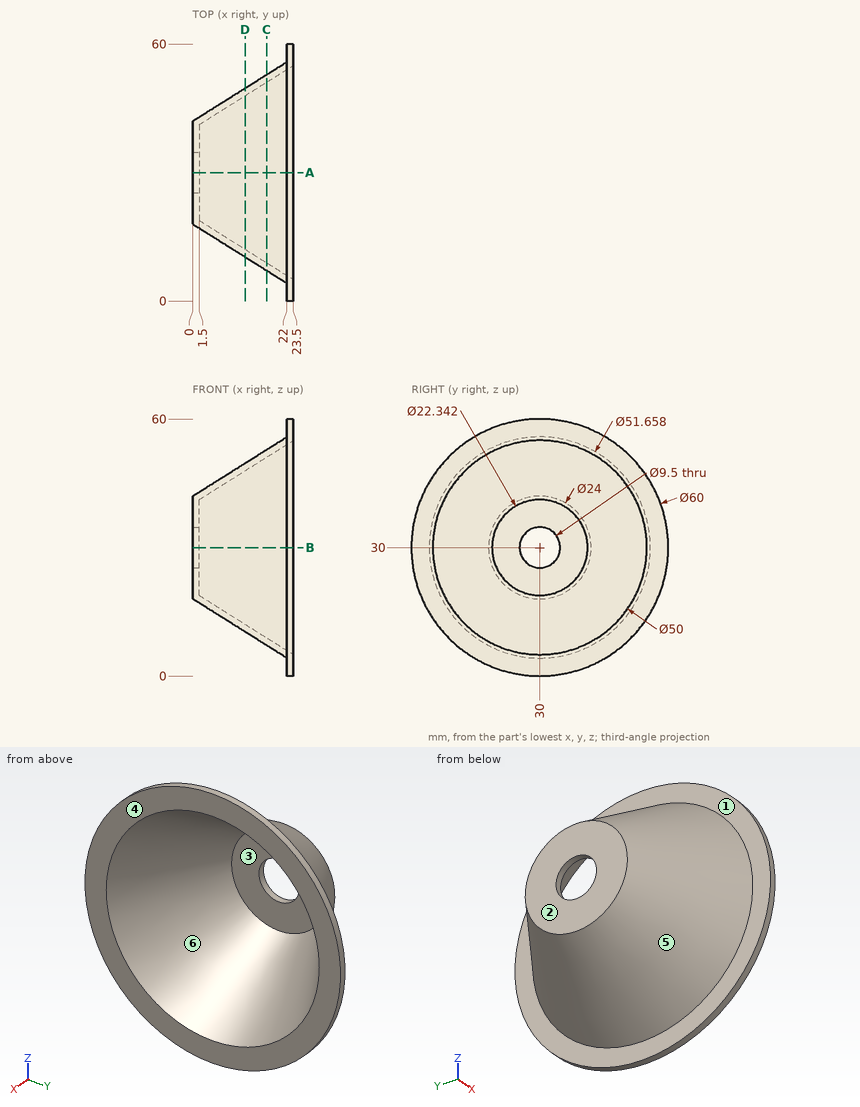
Part print with two shaded views. Sizes in mm from the minimum x, y, z corner. A direction names the side the tool comes from. Coordinates: 2 decimals unless noted, no trailing zeros. Write each loop counter-clockwise with the first axis right and the second up, starting at its lowest first coordinate (ties: lowest second). Pieces come first, ordered by that corner, then holes. Notation, with made-up numbers: (-8, 4) - (14, 4) arc R8 ccw to (14, 14) - close; hole circle Ø1 at (78, -8). An arc over 180 degrees is marked (long way). Use a Markdown table: item, result. Add a question column.
Item 1: Drop flat-ended pins along their axis: pin 1 (10 mm diameter, centred on x = 17.5, y = 52.5, fed in from -Z); pin 2 (12 mm diameter, centred on y = 51.5, z = 10.5, fed in from -X); pin 3 (10 mm diameter, centred on y = 41.5, z = 35, fed in from +X). Give the stop position or say it passes through.
Item 2: Band-saw the part on D-D, the plane x = 12.25. Write the cut outline in (y, z).
Item 3: 3-axis set-ups, long thin cutter, end or side, ignore diameter. For the marked faces 1 and 2: which of +Z, -Z, +X, -X, +Y, -Y reach the whole face in a straight line?
Item 4: Band-saw the part on C-C, the plane x = 17.25. Write the cut outline in (y, z).
Item 5: Drill centre lines: line 1 along X through (y, z) = (48, 8.5); line 2 along Y through (x, z) = (15.5, 24); line 3 along Y through (x, z) = (0.45, 30). Where is each one in solid material? Low to high.
Item 6: Band-saw the part on A-A, the plane y = 30. Write the cut outline in (x, z), and give its area (3 significant figures).
Item 7: Two-plate mould, pull along Z, no slides. Class the marked faces 3, 4, 5 and 6: pulls with the +Z half, pulls with the -Z half, needs draft (parallel to the pull), parting line crosses it, or undercut.
A:
| question | item | result |
|---|---|---|
| 1 | pin 1 | stops at z = 7.93 |
| 1 | pin 2 | stops at x = 17.54 |
| 1 | pin 3 | stops at x = 11.63 |
| 2 | outline | circle Ø39.4 at (30, 30); hole circle Ø35.86 at (30, 30) |
| 3 | face 1 | -X |
| 3 | face 2 | +Z, -Z, -X, +Y, -Y |
| 4 | outline | circle Ø45.69 at (30, 30); hole circle Ø42.14 at (30, 30) |
| 5 | line 1 | x = 22 to 23.5 |
| 5 | line 2 | y = 9.1 to 10.95, 49.05 to 50.9 |
| 5 | line 3 | y = 17.72 to 25.25, 34.75 to 42.28 |
| 6 | outline | (0, 18) - (22, 4.17) - (22, 0) - (23.5, 0) - (23.5, 5) - (1.5, 18.83) - (1.5, 25.25) - (0, 25.25) - close; (0, 34.75) - (1.5, 34.75) - (1.5, 41.17) - (23.5, 55) - (23.5, 60) - (22, 60) - (22, 55.83) - (0, 42) - close |
| 6 | area | 112 mm² |
| 7 | face 3 | undercut |
| 7 | face 4 | needs draft |
| 7 | face 5 | parting line crosses it |
| 7 | face 6 | undercut |
